Build history of the part. All positions in model axes, mm. A direction names the side the tool comes from. Round coordinates to 2 decimals unless told otherwise and drop trailing zeros. Write each loop counter-clockwise with the first axis right and the second up, starting at its lowest first coordinate (ties: lowest second). Pieces come first, ordered by that corner, then holes. Notation, with made-up numbers: (33, 14) - (62, 14) arc R33 cw to (62, 52) - close; hole circle Ø7 at (3.25, 22.25). An arc over 180 degrees is marked (long way). Answer as a JSON object with one key per item and string values. Group by question number.
Item 1: Probe line 1 (Z direction, x = -4.5, y = -2.75); line 2 (Y direction, x = -2.25, z = 3.7); line 3 (X direction, y = -3, z = 2.5). List the from-to ranges inside material, lowest first. Write a range as from..to.
Item 2: Two-plate mould, pull along X, no slides. Class faces 1 (the flat face through (0.09, 3.67, 2.74)), 2 (the flat face through (-5, 1.827, 3)), 3 (the cylindrical face through (-7.493, 0.33, 0.986)), 4 (the flat face through (5.317, 1.01, 2.74)): +X half, -X half, draft (parallel to the pull), parting line (faces both ways), or undercut.
Item 3: Slice it at A-A, the plane y = 1. List the corners of the cut face in (x, z).
Item 4: Which spindle directions (+Z, -Z, +X, -X, +Y, -Y) get a long thin tool onto all of the face, cutting with end or side? Do faces 5 (the cylindrical face through (-1.937, 2.47, 2.986)), 6 (the flat face through (1, 5, 4)). Say none if no direction does.
Item 5: Slice it at C-C, the plane z = 3. Give the number of separate pieces and of enclosed holes in the cut face, then the cut area to 3 significant figures.
Item 6: Slice it at B-B, the plane z = 0.5. List the corners of the cut face in (x, y).
Item 7: Flat gauge pins, fed straight in: pin 1 (6 mm diameter, centred on x = 2, y = 1, fed in from -Z); pin 2 (0.9 mm diameter, centred on y = 0, z = 3, fed in from -X); pin 3 (1 mm diameter, centred on x = 3, z = 3, fed in from -Y); pin 4 (0.7 mm diameter, centred on x = 1.5, y = 4, fed in from +Z). Where does each tip first touch, or does it go through?
from build123d import *

# Parameters (mm, degrees)
F0_R     = 7.5
F1_DEPTH = 2
F2_R     = 1.1
F2_R_2   = 0.70626
F2_R_3   = 0.694508
F3_DEPTH = 2
F5_DEPTH = 1.5


with BuildPart() as f1:
    # F0 (on Top) → F1 (new body)
    with BuildSketch(Plane.XY):
        Circle(F0_R)
    extrude(amount=F1_DEPTH)

    # F2 (on face) → F3 (join)
    with BuildSketch(Plane.XY.offset(2)):
        with BuildLine():
            ThreePointArc((5.709143, -1.852388), (6.202641, 0.241821), (4.239235, -0.638116))
            ThreePointArc((4.239235, -0.638116), (1.796573, -5.09184), (5.709143, -1.852388))
        make_face()
        with BuildLine():
            ThreePointArc((4.765573, -0.876203), (5.884142, -0.14373), (5.375983, -1.380455))
            ThreePointArc((5.375983, -1.380455), (5.090193, -1.104827), (4.765573, -0.876203))
        make_face(mode=Mode.SUBTRACT)
        with Locations((1.537181, 4.217723)):
            Circle(F2_R)
        with Locations((1.537181, 4.217723)):
            Circle(F2_R_2, mode=Mode.SUBTRACT)
        with Locations((4.536864, 2.431652)):
            Circle(F2_R)
        with Locations((4.536864, 2.431652)):
            Circle(F2_R_3, mode=Mode.SUBTRACT)
        with BuildLine():
            Line((-3.205112, 0.120576), (-3.205112, -0.691418))
            ThreePointArc((-3.205112, -0.691418), (-1.455226, -0.020752), (-0.814583, 1.740348))
            ThreePointArc((-0.814583, 1.740348), (-0.263788, 3.372074), (-1.977704, 3.540587))
            ThreePointArc((-1.977704, 3.540587), (-4.098503, 3.56954), (-5.307508, 1.82686))
            Line((-5.307508, 1.82686), (-4.48911, 1.82686))
            ThreePointArc((-4.48911, 1.82686), (-1.908134, 2.43282), (-3.205112, 0.120576))
        make_face()
        with BuildLine():
            ThreePointArc((-1.583388, 3.265403), (-0.658546, 3.117024), (-0.903388, 2.212922))
            ThreePointArc((-0.903388, 2.212922), (-1.168911, 2.787281), (-1.583388, 3.265403))
        make_face(mode=Mode.SUBTRACT)
    extrude(amount=F3_DEPTH)

    # F4 (on face) → F5 (join)
    with BuildSketch(Plane.XY.offset(2)):
        Polygon((1.142579, 4.2306), (-0.998543, 3.087274), (-0.813259, 2.813969), (1.321921, 3.866934), align=None)
        Polygon((4.455775, 2.74566), (1.968617, 4.249523), (1.769449, 3.881378), (4.239448, 2.387889), align=None)
        Polygon((4.908196, 2.244463), (4.531938, 2.055495), (5.313687, -0.303966), (5.709143, -0.172942), align=None)
    extrude(amount=F5_DEPTH)


solid = f1.part
Geometry says:
{
 "1": {"line 1": "z = 0..2", "line 2": "y = -0.54..0.37, 2.76..3.67", "line 3": "x = 0.86..6.03"},
 "2": {"face 1": "undercut", "face 2": "draft", "face 3": "parting line", "face 4": "+X half"},
 "3": {"outline": "(-7.43, 0) - (7.43, 0) - (7.43, 2) - (5.32, 2) - (5.32, 3.5) - (4.88, 3.5) - (4.88, 2) - (-0.88, 2) - (-0.88, 4) - (-1.73, 4) - (-1.73, 2) - (-7.43, 2) - close"},
 "4": {"face 5": "+Z", "face 6": "+Z, +X, -X, +Y, -Y"},
 "5": {"separate pieces": "1", "enclosed holes": "4", "area": "38.2 mm^2"},
 "6": {"outline": "circle Ø15 at (0, 0)"},
 "7": {"pin 1": "stops at z = 0", "pin 2": "stops at x = -3.21", "pin 3": "stops at y = -5.68", "pin 4": "stops at z = 3.5"}
}
